Build history of the part. All positions in model axes, mm. Give positions to 0.01 mm unless a question says otherwise; leave off trailing zeros. Order: outer loops, then holes, each group sorted by start corner. A loop starts at its lowest first (then second) coordinate and runs counter-clockwise, first axis right, second up. Notation, with made-up numbers: (58.25, 84) - (89.25, 84) arc R14 ccw to (89.25, 101) - close; hole circle Ø10 at (-28, -26.75). An arc over 180 degrees is marked (long way). Write each question's results on one line, items separated by ' | '. Start each with the question number.
1) Drill centre lines: line 1 along Z through (x, y) = (0, -23.75); line 2 along Y through (x, z) = (0, 610) (3 decimals); line 3 along Y through (x, z) = (-13.5, 710.5). Where is each one in solid material? Low to high. Write a range as from..to.
2) Cut at B-B on x = 13.5. List the corners of the cut face in (y, z), plus the area to 3 significant figures.
3) Cut at A-A on y = 0. List the corners of the cut face in (x, z) (3 decimals).
4) Two-plate mould, pull along X, no slides. Class faces 1 (the face through (-28.547, 1.256, 450.799)), 2 (the face through (21.199, 6.676, 450.799)), 3 (the face through (15, -17, 914.4)): +X half, -X half, draft (parallel to the pull), parting line (faces both ways), or undercut.
5) Drop flat-ended pins along their axis: pin 1 Ø1.5 at (x, z) = (-12.5, 815.5) entering from -Y; pin 2 Ø3 at (y, z) = (22.5, 478) entering from +X; pin 3 Ø12.5 at (x, z) = (-3.175, 38.1) entering from -Y (3 decimals); pin 4 Ø4 at (x, z) = (-7.5, 169) entering from +Y. Give the stop position or say it passes through.
6) Cut at C-C on z = 558. List the corners of the cut face in (x, y) (3 decimals).
from build123d import *

# Parameters (mm, degrees)
SKETCH1_R           = 28.575
SKETCH1_R_2         = 22.225
BOSS_EXTRUDE1_DEPTH = 914.4
SKETCH2_R           = 4.7625
CUT_EXTRUDE1_DEPTH  = 916.292533155


with BuildPart() as part:
    # Sketch1 → Boss-Extrude1 (new body)
    with BuildSketch(Plane.XY):
        Circle(SKETCH1_R)
        Circle(SKETCH1_R_2, mode=Mode.SUBTRACT)
    extrude(amount=BOSS_EXTRUDE1_DEPTH)

    # Sketch2 → Cut-Extrude1 (cut, through all)
    with BuildSketch(Plane(origin=(0, 0, 0), x_dir=(1, 0, 0), z_dir=(0, 1, 0))):
        with Locations(Location((-3.175, -38.1, 0), (0, 0, 270))):
            Circle(SKETCH2_R)
        with Locations(Location((-0.006183063, -88.801070987, 0), (0, 0, 270))):
            Circle(SKETCH2_R)
        with Locations(Location((0, -876.3, 0), (0, 0, 270))):
            Circle(SKETCH2_R)
        with Locations(Location((0, -825.5, 0), (0, 0, 270))):
            Circle(SKETCH2_R)
    extrude(amount=-CUT_EXTRUDE1_DEPTH, mode=Mode.SUBTRACT)


solid = part.part
Results:
1) line 1: 0..34.55, 41.65..84.04, 93.56..820.74, 830.26..871.54, 881.06..914.4 | line 2: -28.575..-22.225, 22.225..28.575 | line 3: -25.18..-17.66, 17.66..25.18
2) outline: (-25.18, 0) - (-17.66, 0) - (-17.66, 914.4) - (-25.18, 914.4) - close; (17.66, 0) - (25.18, 0) - (25.18, 914.4) - (17.66, 914.4) - close | area: 13,800 mm^2
3) outline: (-28.575, 0) - (-22.225, 0) - (-22.225, 914.4) - (-28.575, 914.4) - close; (22.225, 0) - (28.575, 0) - (28.575, 914.4) - (22.225, 914.4) - close
4) face 1: parting line | face 2: undercut | face 3: draft
5) pin 1: y = -26.05 | pin 2: x = 19.38 | pin 3: y = -28.575 | pin 4: y = 28.04
6) outline: circle Ø57.15 at (0, 0); hole circle Ø44.45 at (0, 0)
